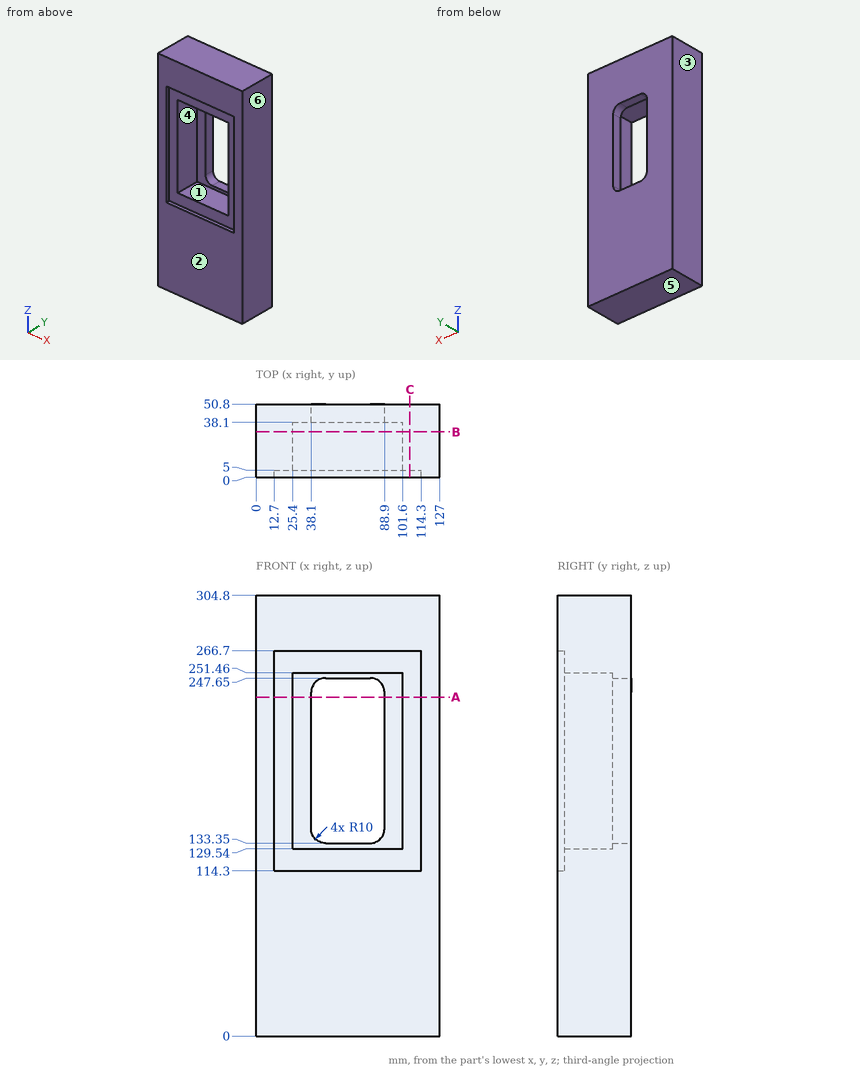
Check sheet for the drawn part. Datum: minimum x, y, z corner. Units: mm. A direction names the side the tool comes from. Give positions to 0.01 mm unless a question says otherwise; leave off trailing zeros. Write each loop counter-clockwise with the first axis right and the second up, starting at its lowest first coordinate (ties: lowest second). Pieces come first, ordered by that corner, then holes. Notation, with made-up numbers: (83.5, 22) -> (129.5, 22) arc R12 ccw to (129.5, 45) -> close; hole circle Ø2 at (38, 47.25). An arc over 180 degrees is marked (long way). Use one line per item in the form item = value. Start each with the question number.
1. Mould release check, pull along X, two halves, no side actions. Record for the marked faces 3, 4, 5 and 6: pulls with the +X half, pulls with the -X half, needs draft (parallel to the pull), parting line crosses it, or undercut.
2. Section check B-B (y = 31.5). Record the cut outline in (x, z).
3. Thickness scan on line 1 along X through (y, z) = (13, 192); line 2 along Z through (x, y) = (79.5, 48.5); line 3 along Z through (x, y) = (52.5, 19). Record the ranges inside material, lowest first. Write a range as from..to.
4. Section check C-C (x = 106.5). Record the cut outline in (y, z).
5. Access from +Z, -Z, +X, -X, +Y, -Y to the whole of each face (thin tool, end or side, straight path). Record for the marked faces 1 and 2.
6. Section check A-A (z = 234.5). Record the cut outline in (x, y).
Conclusion:
q1.face_3 = pulls with the -X half
q1.face_4 = undercut
q1.face_5 = needs draft
q1.face_6 = pulls with the +X half
q2.outline = (0, 0) -> (127, 0) -> (127, 304.8) -> (0, 304.8) -> close; hole (25.4, 129.54) -> (101.6, 129.54) -> (101.6, 251.46) -> (25.4, 251.46) -> close
q3.line_1 = 0..25.4, 101.6..127
q3.line_2 = 0..133.37, 247.63..304.8
q3.line_3 = 0..129.54, 251.46..304.8
q4.outline = (0, 0) -> (50.8, 0) -> (50.8, 304.8) -> (0, 304.8) -> (0, 266.7) -> (5, 266.7) -> (5, 114.3) -> (0, 114.3) -> close
q5.face_1 = -Y
q5.face_2 = +Z, -Z, +X, -X, -Y
q6.outline = (0, 0) -> (12.7, 0) -> (12.7, 5) -> (25.4, 5) -> (25.4, 38.1) -> (38.1, 38.1) -> (38.1, 50.8) -> (0, 50.8) -> close; (88.9, 38.1) -> (101.6, 38.1) -> (101.6, 5) -> (114.3, 5) -> (114.3, 0) -> (127, 0) -> (127, 50.8) -> (88.9, 50.8) -> close
